Could you check a few things on this model? Use its own coordinates, in mm. A direction names the side the tool comes from. Give positions to 0.01 mm unless a question says otherwise; leave off trailing zeros. Write each loop counter-clockwise with the first axis right and the second up, starting at its lowest first coordinate (ties: lowest second). Pieces come first, ordered by that corner, then holes. Notation, with made-up numbers: M 58.5,36.5 L 88.5,36.5 A22 ccw 88.5,55.5 Z; hole C 82.25,83 d10. An arc over 180 degrees is marked long. One line per item, written item: value.
```python
from build123d import *

# Parameters (mm, degrees)
SKETCH_1_R          = 23
EXTRUDE_1_DEPTH     = 20
SKETCH_2_R          = 21
CUT_EXTRUDE_1_DEPTH = 18
EXTRUDE_START       = -20
EXTRUDE_2_DEPTH     = 20
FILLET_1_R          = 3
SKETCH_6_R          = 21
CUT_EXTRUDE_2_DEPTH = 18
CUT_EXTRUDE_START   = -4
SKETCH_7_R          = 3.25
CUT_EXTRUDE_3_DEPTH = 4
FILLET_START        = 16
FILLET_2_DEPTH      = 4
CUT_EXTRUDE_4_REACH = 41.58


with BuildPart() as part:
    # Эскиз1 → Бобышка-Вытянуть1 (new body)
    with BuildSketch(Plane.XY):
        Circle(SKETCH_1_R)
    extrude(amount=EXTRUDE_1_DEPTH)

    # Эскиз2 → Вырез-Вытянуть1 (cut)
    with BuildSketch(Plane.XY.offset(20)):
        Circle(SKETCH_2_R)
    extrude(amount=-CUT_EXTRUDE_1_DEPTH, mode=Mode.SUBTRACT)

    # Эскиз5 → Бобышка-Вытянуть2 (add)
    with BuildSketch(Plane.XY.offset(20).offset(EXTRUDE_START)):
        with BuildLine():
            ThreePointArc((-13.428172595, 16.145717103), (-18.764406843, 16.895547811), (-17.460895421, 11.666924663))
            ThreePointArc((-17.460895421, 11.666924663), (-19.605188956, 7.52572694), (-20.782670455, 3.013404848))
            ThreePointArc((-20.782670455, 3.013404848), (-25.25, 0), (-20.782670455, -3.013404848))
            ThreePointArc((-20.782670455, -3.013404848), (-19.605188956, -7.52572694), (-17.460895421, -11.666924663))
            ThreePointArc((-17.460895421, -11.666924663), (-18.764406843, -16.895547811), (-13.428172595, -16.145717103))
            ThreePointArc((-13.428172595, -16.145717103), (0, -21), (13.428172595, -16.145717103))
            ThreePointArc((13.428172595, -16.145717103), (18.764406843, -16.895547811), (17.460895421, -11.666924663))
            ThreePointArc((17.460895421, -11.666924663), (21, 0), (17.460895421, 11.666924663))
            ThreePointArc((17.460895421, 11.666924663), (18.764406843, 16.895547811), (13.428172595, 16.145717103))
            ThreePointArc((13.428172595, 16.145717103), (0, 21), (-13.428172595, 16.145717103))
        make_face()
    extrude(amount=EXTRUDE_2_DEPTH)

    # Скругление1
    fillet_1_edges = [part.edges().sort_by_distance(p)[0] for p in [
        (19.041496109, 12.900442858, 10),
        (14.820151209, -17.588721334, 10),
        (-19.041496109, -12.900442858, 10),
        (-22.782670455, 3.154350481, 10),
        (-14.820151209, 17.588721334, 10),
        (14.820151209, 17.588721334, 10),
        (19.041496109, -12.900442858, 10),
        (-14.820151209, -17.588721334, 10),
        (-22.782670455, -3.154350481, 10),
        (-19.041496109, 12.900442858, 10),
    ]]
    fillet(fillet_1_edges, radius=FILLET_1_R)

    # Эскиз6 → Вырез-Вытянуть2 (cut)
    with BuildSketch(Plane.XY.offset(20)):
        Circle(SKETCH_6_R)
    extrude(amount=-CUT_EXTRUDE_2_DEPTH, mode=Mode.SUBTRACT)

    # Эскиз7 → Вырез-Вытянуть3 (cut)
    with BuildSketch(Plane.XY.offset(20).offset(CUT_EXTRUDE_START)):
        with Locations((-16.349186161, 14.72087334)):
            Circle(SKETCH_7_R)
        with Locations((16.349186161, 14.72087334)):
            Circle(SKETCH_7_R)
        with Locations((-16.349186161, -14.72087334)):
            Circle(SKETCH_7_R)
        with Locations((-22, 0)):
            Circle(SKETCH_7_R)
        with Locations((16.349186161, -14.72087334)):
            Circle(SKETCH_7_R)
    extrude(amount=CUT_EXTRUDE_3_DEPTH, mode=Mode.SUBTRACT)

    # Скругление2: read off the stored shape, not the designer's step
    # Скругление2 outline → Скругление2 (cut)
    with BuildSketch(Plane.XY.offset(FILLET_START)):
        with BuildLine():
            ThreePointArc((-13.776491508, -18.421379011), (-14.209607213, -17.709819826), (-13.95357615, -16.917132131))
            ThreePointArc((-13.95357615, -16.917132131), (-14.831000199, -17.59447933), (-15.885025704, -17.937557202))
            ThreePointArc((-15.885025704, -17.937557202), (-14.785629767, -17.982793014), (-13.776491508, -18.421379011))
        make_face()
        with BuildLine():
            ThreePointArc((-19.499730713, -13.923020582), (-19.048356591, -12.910630542), (-18.283004183, -12.108815175))
            ThreePointArc((-18.283004183, -12.108815175), (-19.098111986, -12.280585247), (-19.760500256, -11.775464006))
            ThreePointArc((-19.760500256, -11.775464006), (-19.42980055, -12.824918821), (-19.499730713, -13.923020582))
        make_face()
        with BuildLine():
            ThreePointArc((-22.564236885, -4.471480374), (-22.409978551, -3.652877874), (-21.689298793, -3.235114335))
            ThreePointArc((-21.689298793, -3.235114335), (-22.794585678, -3.151370115), (-23.807443182, -2.701045935))
            ThreePointArc((-23.807443182, -2.701045935), (-23.020701446, -3.470302164), (-22.564236885, -4.471480374))
        make_face()
        with BuildLine():
            ThreePointArc((-23.807443182, 2.701045935), (-22.794585678, 3.151370115), (-21.689298793, 3.235114335))
            ThreePointArc((-21.689298793, 3.235114335), (-22.409978551, 3.652877874), (-22.564236885, 4.471480374))
            ThreePointArc((-22.564236885, 4.471480374), (-23.020701446, 3.470302164), (-23.807443182, 2.701045935))
        make_face()
        with BuildLine():
            ThreePointArc((-19.760500256, 11.775464006), (-19.098111986, 12.280585247), (-18.283004183, 12.108815175))
            ThreePointArc((-18.283004183, 12.108815175), (-19.048356591, 12.910630542), (-19.499730713, 13.923020582))
            ThreePointArc((-19.499730713, 13.923020582), (-19.42980055, 12.824918821), (-19.760500256, 11.775464006))
        make_face()
        with BuildLine():
            ThreePointArc((-15.885025704, 17.937557202), (-14.831000199, 17.59447933), (-13.95357615, 16.917132131))
            ThreePointArc((-13.95357615, 16.917132131), (-14.209607213, 17.709819826), (-13.776491508, 18.421379011))
            ThreePointArc((-13.776491508, 18.421379011), (-14.785629767, 17.982793014), (-15.885025704, 17.937557202))
        make_face()
        with BuildLine():
            ThreePointArc((13.776491508, 18.421379011), (14.209607213, 17.709819826), (13.95357615, 16.917132131))
            ThreePointArc((13.95357615, 16.917132131), (14.831000199, 17.59447933), (15.885025704, 17.937557202))
            ThreePointArc((15.885025704, 17.937557202), (14.785629767, 17.982793014), (13.776491508, 18.421379011))
        make_face()
        with BuildLine():
            ThreePointArc((19.499730713, 13.923020582), (19.048356591, 12.910630542), (18.283004183, 12.108815175))
            ThreePointArc((18.283004183, 12.108815175), (19.098111986, 12.280585247), (19.760500256, 11.775464006))
            ThreePointArc((19.760500256, 11.775464006), (19.42980055, 12.824918821), (19.499730713, 13.923020582))
        make_face()
        with BuildLine():
            ThreePointArc((19.760500256, -11.775464006), (19.098111986, -12.280585247), (18.283004183, -12.108815175))
            ThreePointArc((18.283004183, -12.108815175), (19.048356591, -12.910630542), (19.499730713, -13.923020582))
            ThreePointArc((19.499730713, -13.923020582), (19.42980055, -12.824918821), (19.760500256, -11.775464006))
        make_face()
        with BuildLine():
            ThreePointArc((15.885025704, -17.937557202), (14.831000199, -17.59447933), (13.95357615, -16.917132131))
            ThreePointArc((13.95357615, -16.917132131), (14.209607213, -17.709819826), (13.776491508, -18.421379011))
            ThreePointArc((13.776491508, -18.421379011), (14.785629767, -17.982793014), (15.885025704, -17.937557202))
        make_face()
        with BuildLine():
            ThreePointArc((-13.951391744, -16.914747069), (-13.306228642, -16.594083591), (-12.612990263, -16.790249451))
            ThreePointArc((-12.612990263, -16.790249451), (-13.024568946, -16.473026551), (-13.428172595, -16.145717103))
            ThreePointArc((-13.428172595, -16.145717103), (-13.662128037, -16.549046921), (-13.951391744, -16.914747069))
        make_face()
        with BuildLine():
            ThreePointArc((13.428172595, -16.145717103), (13.024568946, -16.473026551), (12.612990263, -16.790249451))
            ThreePointArc((12.612990263, -16.790249451), (13.306228642, -16.594083591), (13.951391744, -16.914747069))
            ThreePointArc((13.951391744, -16.914747069), (13.662128037, -16.549046921), (13.428172595, -16.145717103))
        make_face()
        with BuildLine():
            ThreePointArc((-18.280403854, -12.106892043), (-17.886470759, -11.857439027), (-17.460895421, -11.666924663))
            ThreePointArc((-17.460895421, -11.666924663), (-17.744223765, -11.231318844), (-18.016687197, -10.78883601))
            ThreePointArc((-18.016687197, -10.78883601), (-17.894059096, -11.498781672), (-18.280403854, -12.106892043))
        make_face()
        with BuildLine():
            ThreePointArc((18.016687197, -10.78883601), (17.744223765, -11.231318844), (17.460895421, -11.666924663))
            ThreePointArc((17.460895421, -11.666924663), (17.886470759, -11.857439027), (18.280403854, -12.106892043))
            ThreePointArc((18.280403854, -12.106892043), (17.894059096, -11.498781672), (18.016687197, -10.78883601))
        make_face()
        with BuildLine():
            ThreePointArc((-21.686079545, -3.234803541), (-20.992064177, -3.428202514), (-20.608148244, -4.037849175))
            ThreePointArc((-20.608148244, -4.037849175), (-20.701747261, -3.526706725), (-20.782670455, -3.013404848))
            ThreePointArc((-20.782670455, -3.013404848), (-21.226413556, -3.156590568), (-21.686079545, -3.234803541))
        make_face()
        with BuildLine():
            ThreePointArc((-21.686079545, 3.234803541), (-21.226413556, 3.156590568), (-20.782670455, 3.013404848))
            ThreePointArc((-20.782670455, 3.013404848), (-20.701747261, 3.526706725), (-20.608148244, 4.037849175))
            ThreePointArc((-20.608148244, 4.037849175), (-20.992064177, 3.428202514), (-21.686079545, 3.234803541))
        make_face()
        with BuildLine():
            ThreePointArc((17.460895421, 11.666924663), (17.744223765, 11.231318844), (18.016687197, 10.78883601))
            ThreePointArc((18.016687197, 10.78883601), (17.894059096, 11.498781672), (18.280403854, 12.106892043))
            ThreePointArc((18.280403854, 12.106892043), (17.886470759, 11.857439027), (17.460895421, 11.666924663))
        make_face()
        with BuildLine():
            ThreePointArc((-18.280403854, 12.106892043), (-17.894059096, 11.498781672), (-18.016687197, 10.78883601))
            ThreePointArc((-18.016687197, 10.78883601), (-17.744223765, 11.231318844), (-17.460895421, 11.666924663))
            ThreePointArc((-17.460895421, 11.666924663), (-17.886470759, 11.857439027), (-18.280403854, 12.106892043))
        make_face()
        with BuildLine():
            ThreePointArc((12.612990263, 16.790249451), (13.024568946, 16.473026551), (13.428172595, 16.145717103))
            ThreePointArc((13.428172595, 16.145717103), (13.662128037, 16.549046921), (13.951391744, 16.914747069))
            ThreePointArc((13.951391744, 16.914747069), (13.306228642, 16.594083591), (12.612990263, 16.790249451))
        make_face()
        with BuildLine():
            ThreePointArc((-13.951391744, 16.914747069), (-13.662128037, 16.549046921), (-13.428172595, 16.145717103))
            ThreePointArc((-13.428172595, 16.145717103), (-13.024568946, 16.473026551), (-12.612990263, 16.790249451))
            ThreePointArc((-12.612990263, 16.790249451), (-13.306228642, 16.594083591), (-13.951391744, 16.914747069))
        make_face()
    extrude(amount=FILLET_2_DEPTH, mode=Mode.SUBTRACT)

    # Эскиз8 → Вырез-Вытянуть4 (cut, up to next)
    with BuildSketch(Plane(origin=(0, 0, 0), x_dir=(-1, 0, 0), z_dir=(0, 0, -1)), mode=Mode.PRIVATE) as cut_extrude_4_sk1:
        with BuildLine():
            ThreePointArc((-15.885025704, 17.937557202), (-18.764406843, 16.895547811), (-19.499730713, 13.923020582))
            ThreePointArc((-19.499730713, 13.923020582), (-19.438094361, 12.762156961), (-19.822395798, 11.665017138))
            ThreePointArc((-19.822395798, 11.665017138), (-17.092330986, 15.390003946), (-13.673119525, 18.494480324))
            ThreePointArc((-13.673119525, 18.494480324), (-14.724078663, 17.997601791), (-15.885025704, 17.937557202))
        make_face()
    cut_extrude_4_tool1 = extrude(cut_extrude_4_sk1.sketch, amount=-CUT_EXTRUDE_4_REACH, mode=Mode.PRIVATE) & part.part
    add(cut_extrude_4_tool1.solids().sort_by_distance((17.719386, 15.954607, 0))[0], mode=Mode.SUBTRACT)


solid = part.part
```
1) We'd pull the mould along Y, two halves only. Please class faces 1 (the face through (-23, 0, 16)), 2 (the face through (-25.25, 0.04, 7.89)), 3 (the face through (-0.1, 21.5, 20)): pulls with the +Y half, pulls with the -Y half, needs draft (parallel to the pull), parting line crosses it, or undercut.
Outcome:
face 1: undercut
face 2: parting line crosses it
face 3: needs draft
2) If we section it at C-C, the plane z = 17.25: Give the number of separate pieces and of enclosed holes in the cut face, then the cut area to 3 significant figures.
Outcome:
separate pieces: 5
enclosed holes: 0
area: 207 mm^2
3) If we section it at A-A, the plane x = 0: Write out the boundary of the cut face in (y, z).
Outcome:
outline: M -23,0 L 23,0 L 23,20 L 21,20 L 21,2 L -21,2 L -21,20 L -23,20 Z
4) On a 3-axis mill with a long thin cutter (end or side, diameter ignored), from which of +Z, -Z, +X, -X, +Y, -Y can I reach the whole of each face in a straight line? I mean faces 4 (the face through (-19.086, -12.283, 17.972)), 5 (the face through (13.316, 16.595, 17.972)), 6 (the face through (14.215, 17.649, 17.972)), 7 (the face through (-22.417, -3.663, 17.972)). Say none if no direction works.
Outcome:
face 4: +Z, -Y
face 5: +Z
face 6: +Z, +X
face 7: +Z, -X
5) If we section it at B-B, the plane y = 0: Write out the boundary of the cut face in (x, z), then the cut area to 3 significant figures.
Outcome:
outline: M -25.25,0 L 23,0 L 23,20 L 21,20 L 21,2 L -21,2 L -21,16 L -25.25,16 Z
area: 192 mm^2
6) I'm going to push flat-ended pins straight in: pin 1 (8 mm diameter, centred on x = 2.5, z = 10.5, fed in from -Y); pin 2 (12 mm diameter, centred on y = 12, z = 5.5, fed in from +X); pin 3 (3 mm diameter, centred on y = 7, z = 5.5, fed in from -X). Where does each tip first touch, or does it pass through?
Outcome:
pin 1: stops at y = -23
pin 2: stops at x = 22.2
pin 3: stops at x = -22.33
7) Please list where these lines run through material, in increasing order: L1, parallel to Y at x = 0, z = 15; L2, parallel to Z at x = -5, y = -2.5; L3, parallel to X at y = 4, z = 3.5. Write a range as from..to.
Outcome:
L1: y = -23..-21, 21..23
L2: z = 0..2
L3: x = -22.72..-20.62, 20.62..22.65
